```python
from build123d import *

# Parameters (mm, degrees)
BOSS_EXTRUDE1_DEPTH = 10
SKETCH1_3_R         = 234
SKETCH1_3_R_2       = 224
BOSS_EXTRUDE2_DEPTH = 10


with BuildPart() as part:
    # Sketch1 → Boss-Extrude1 (new body)
    with BuildSketch(Plane(origin=(0, 0, 0), x_dir=(1, 0, 0), z_dir=(0, 1, 0))):
        Polygon((514.396103797, 270), (0, 270), (-325.603896203, 270), (-325.603896203, -270), (514.396103797, -270), align=None)
        Polygon((-65, -200), (-65, 200), (0, 200), (65, 200), (65, -200), align=None, mode=Mode.SUBTRACT)
    extrude(amount=-BOSS_EXTRUDE1_DEPTH)

    # Sketch1_3 → Boss-Extrude2 (add)
    with BuildSketch(Plane(origin=(0, 0, 0), x_dir=(1, 0, 0), z_dir=(0, 1, 0))):
        with Locations(Location((0, 0, 0), (0, 0, 270))):
            Circle(SKETCH1_3_R)
        with Locations(Location((0, 0, 0), (0, 0, 270))):
            Circle(SKETCH1_3_R_2, mode=Mode.SUBTRACT)
    extrude(amount=BOSS_EXTRUDE2_DEPTH)


solid = part.part
```
Geometry check sheet. Reference: the model listing, model coordinates, mm. A direction names the side the tool comes from. Round coordinates to 2 decimals unless told otherwise and drop trailing zeros. Order: outer loops, then holes, each group sorted by start corner. A loop starts at its lowest first (then second) coordinate and runs counter-clockwise, first axis right, second up. Notation, with made-up numbers: M -34.75,-30 L 0.25,-30 A35 ccw 0.25,8 Z; hole C 62.5,-23 d9. An arc over 180 degrees is marked long. Write item = value, one per line.
Q1. Set-up check for faces 4 (the flat face through (89, -10, -4)), 5 (the flat face through (96, 0, -3)): record each of +Z, -Z, +X, -X, +Y, -Y from which the full face is reachable in a straight line by a thin tool's end or side.
Answer block:
face_4 = +Z, -Z, +X, -X, -Y
face_5 = +Y
Q2. Section check C-C (y = -4.5). Enter the section's corners in (x, z), plus the area to 3 significant figures.
Answer block:
outline = M -325.6,-270 L 514.4,-270 L 514.4,270 L -325.6,270 Z; hole M -65,-200 L 65,-200 L 65,200 L -65,200 Z
area = 402,000 mm^2
Q3. Scan lines: line 1 (Z direction, x = 27, y = -1.5); line 2 (X direction, y = -2.25, z = -155); line 3 (X direction, y = 3, z = 0). Record each from-to range of solid material in increasing order.
Answer block:
line_1 = -270 to -200, 200 to 270
line_2 = -325.6 to -65, 65 to 514.4
line_3 = -234 to -224, 224 to 234
Q4. Section check A-A (x = 0). Enter the section's corners in (y, z), plus the area to 3 significant figures.
Answer block:
outline = M -10,-270 L 0,-270 L 0,-234 L 10,-234 L 10,-224 L 0,-224 L 0,-200 L -10,-200 Z; M -10,200 L 0,200 L 0,224 L 10,224 L 10,234 L 0,234 L 0,270 L -10,270 Z
area = 1,600 mm^2
Q5. Release check for a two-part mould opening along X. For faces 1 (the cylindrical face through (-218.673, 4.93, -48.559)), 2 (the cylindrical face through (70.287, 4.93, 223.194)), 3 (the flat face through (-120, 10, 190)) record: released by +X, released by -X, zero draft, split by the parting line, or undercut.
Answer block:
face_1 = undercut
face_2 = split by the parting line
face_3 = zero draft
Q6. Depth check by flat-ended pin: pin 1 Ø8 at (x, z) = (-162.5, 15.5) entering from +Y; pin 2 Ø1 at (y, z) = (2, 34) entering from -X; pin 3 Ø12 at (y, z) = (7.5, -90) entering from -X. Enter the tip coordinate at first touch or a pass-through.
Answer block:
pin_1 = 0
pin_2 = -231.59
pin_3 = -218.4
Q7. Section check D-D (x = 102.5). Enter the section's corners in (y, z).
Answer block:
outline = M -10,-270 L 0,-270 L 0,-210.36 L 10,-210.36 L 10,-199.17 L 0,-199.17 L 0,199.17 L 10,199.17 L 10,210.36 L 0,210.36 L 0,270 L -10,270 Z
Q8. Section check B-B (z = 0). Enter the section's corners in (x, y).
Answer block:
outline = M -325.6,-10 L -65,-10 L -65,0 L -224,0 L -224,10 L -234,10 L -234,0 L -325.6,0 Z; M 65,-10 L 514.4,-10 L 514.4,0 L 234,0 L 234,10 L 224,10 L 224,0 L 65,0 Z
